Part model, mm, in its own coordinate system. Give positions to 0.01 mm unless a question says otherwise; leave off trailing zeros. Write each loop counter-clockwise with the first axis right and the second up, starting at its lowest first coordinate (ties: lowest second). Pieces come first, ordered by that corner, then holes.
```python
from build123d import *

# Parameters (mm, degrees)
SKETCH_W      = 91.28
SKETCH_H      = 58.2
SKETCH_R      = 1.5
SKETCH_R_2    = 2.75
PAD_DEPTH     = 3
SKETCH001_R   = 5
SKETCH001_R_2 = 2.75
PAD001_DEPTH  = 4


with BuildPart() as part:
    # Sketch → Pad (new body)
    with BuildSketch(Plane.XY):
        with Locations((39.34, -24.1)):
            Rectangle(SKETCH_W, SKETCH_H)
        Circle(SKETCH_R, mode=Mode.SUBTRACT)
        with Locations((-1.3, -48.2)):
            Circle(SKETCH_R, mode=Mode.SUBTRACT)
        with Locations((74.9, 0)):
            Circle(SKETCH_R, mode=Mode.SUBTRACT)
        with Locations((79.98, -48.2)):
            Circle(SKETCH_R, mode=Mode.SUBTRACT)
        with Locations((10, -10)):
            Circle(SKETCH_R_2, mode=Mode.SUBTRACT)
        with Locations((70, -10)):
            Circle(SKETCH_R_2, mode=Mode.SUBTRACT)
        with Locations((70, -40)):
            Circle(SKETCH_R_2, mode=Mode.SUBTRACT)
        with Locations((10, -40)):
            Circle(SKETCH_R_2, mode=Mode.SUBTRACT)
    extrude(amount=PAD_DEPTH)

    # Sketch001 → Pad001 (join)
    with BuildSketch(Plane.XY):
        with Locations((10, -10)):
            Circle(SKETCH001_R)
        with Locations((10, -10)):
            Circle(SKETCH001_R_2, mode=Mode.SUBTRACT)
        with Locations((70, -10)):
            Circle(SKETCH001_R)
        with Locations((70, -10)):
            Circle(SKETCH001_R_2, mode=Mode.SUBTRACT)
        with Locations((70, -40)):
            Circle(SKETCH001_R)
        with Locations((70, -40)):
            Circle(SKETCH001_R_2, mode=Mode.SUBTRACT)
        with Locations((10, -40)):
            Circle(SKETCH001_R)
        with Locations((10, -40)):
            Circle(SKETCH001_R_2, mode=Mode.SUBTRACT)
    extrude(amount=-PAD001_DEPTH)


solid = part.part
```
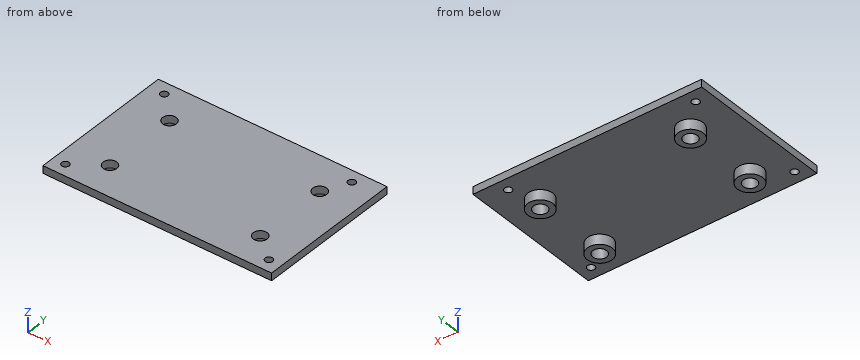
1) Wall check: L1, parallel to Y at x = 10, z = -0.9; L2, parallel to Y at x = 70, z = 1.5; L3, parallel to X at y = -7.5, z = -3.25. Give the ranges that are in metal, low to high.
Answers follow:
L1: y = -45 to -42.75, -37.25 to -35, -15 to -12.75, -7.25 to -5
L2: y = -53.2 to -42.75, -37.25 to -12.75, -7.25 to 5
L3: x = 5.67 to 8.85, 11.15 to 14.33, 65.67 to 68.85, 71.15 to 74.33
2) Saw through at B-B, the plane x = 79.98. Write the cut outline in (y, z).
Answers follow:
outline: (-53.2, 0) - (-49.7, 0) - (-49.7, 3) - (-53.2, 3) - close; (-46.7, 0) - (5, 0) - (5, 3) - (-46.7, 3) - close
3) Saw through at A-A, the plane z = -2.5. Write the cut outline in (x, y).
Answers follow:
outline: circle Ø10 at (10, -40); circle Ø10 at (10, -10); circle Ø10 at (70, -40); circle Ø10 at (70, -10); hole circle Ø5.5 at (10, -40); hole circle Ø5.5 at (10, -10); hole circle Ø5.5 at (70, -40); hole circle Ø5.5 at (70, -10)
4) Saw through at D-D, the plane x = 70. Write the cut outline in (y, z), then the cut area to 3 significant figures.
Answers follow:
outline: (-53.2, 0) - (-45, 0) - (-45, -4) - (-42.75, -4) - (-42.75, 3) - (-53.2, 3) - close; (-37.25, -4) - (-35, -4) - (-35, 0) - (-15, 0) - (-15, -4) - (-12.75, -4) - (-12.75, 3) - (-37.25, 3) - close; (-7.25, -4) - (-5, -4) - (-5, 0) - (5, 0) - (5, 3) - (-7.25, 3) - close
area: 178 mm2
5) Saw through at C-C, the plane y = -10. Write the cut outline in (x, z).
Answers follow:
outline: (-6.3, 0) - (5, 0) - (5, -4) - (7.25, -4) - (7.25, 3) - (-6.3, 3) - close; (12.75, -4) - (15, -4) - (15, 0) - (65, 0) - (65, -4) - (67.25, -4) - (67.25, 3) - (12.75, 3) - close; (72.75, -4) - (75, -4) - (75, 0) - (84.98, 0) - (84.98, 3) - (72.75, 3) - close
6) Pin check, flat tip, straight feed: pin 1 Ø1.8 at (x, y) = (74.9, 0) entering from -Z. Stop position of the tip, or through.
Answers follow:
pin 1: passes through
